from build123d import *

# Parameters (mm, degrees)
SKETCH013_W          = 32
SKETCH013_H          = 3
POCKET_DEPTH         = 6.001
POCKET_DEPTH_BACK    = -6.001
POCKET001_DEPTH      = 6.001
POCKET001_DEPTH_BACK = -6.001
POCKET002_DEPTH      = 6.001
POCKET002_DEPTH_BACK = -6.001


with BuildPart() as part:
    # AdditivePipe: sweep along a path in Sketch
    with BuildLine(Plane.XY) as additivepipe_path:
        ThreePointArc((0, 0), (-10.865453, 68.601773), (-42.398227, 130.488326))
    # Sketch002 → AdditivePipe (sweep)
    with BuildSketch(Plane.XZ):
        Polygon((-20, 6), (-20, -6), (-16, -6), (-16, -3), (-9, -3), (9, -3), (16, -3), (16, -6), (20, -6), (20, 6), (16, 6), (16, 3), (9, 3), (-9, 3), (-16, 3), (-16, 6), align=None)
    sweep(path=additivepipe_path.line)

    # AdditivePipe001: sweep along a path in Sketch001
    with BuildLine(Plane.XY) as additivepipe001_path:
        ThreePointArc((42.398227, 130.488326), (10.865453, 68.601773), (0, 0))
    # Sketch002 → AdditivePipe001 (sweep)
    with BuildSketch(Plane.XZ):
        Polygon((-20, 6), (-20, -6), (-16, -6), (-16, -3), (-9, -3), (9, -3), (16, -3), (16, -6), (20, -6), (20, 6), (16, 6), (16, 3), (9, 3), (-9, 3), (-16, 3), (-16, 6), align=None)
    sweep(path=additivepipe001_path.line)

    # SubtractivePipe: sweep along a path in Sketch
    with BuildLine(Plane.XY) as subtractivepipe_path:
        ThreePointArc((0, 0), (-10.865453, 68.601773), (-42.398227, 130.488326))
    # Sketch013 (on Face1 of AdditivePipe001) → SubtractivePipe (sweep, cut)
    with BuildSketch(Plane.XZ):
        with Locations((0, 4.5)):
            Rectangle(SKETCH013_W, SKETCH013_H)
    subtractivepipe = sweep(path=subtractivepipe_path.line, mode=Mode.SUBTRACT)

    # SubtractivePipe001: sweep along a path in Sketch001
    with BuildLine(Plane.XY) as subtractivepipe001_path:
        ThreePointArc((42.398227, 130.488326), (10.865453, 68.601773), (0, 0))
    # Sketch013 (on Face1 of AdditivePipe001) → SubtractivePipe001 (sweep, cut)
    with BuildSketch(Plane.XZ):
        with Locations((0, 4.5)):
            Rectangle(SKETCH013_W, SKETCH013_H)
    subtractivepipe001 = sweep(path=subtractivepipe001_path.line, mode=Mode.SUBTRACT)

    # Mirrored: SubtractivePipe across XY
    add(subtractivepipe.mirror(Plane.XY), mode=Mode.SUBTRACT)

    # Mirrored001: SubtractivePipe001 across XY
    add(subtractivepipe001.mirror(Plane.XY), mode=Mode.SUBTRACT)

    # Sketch007 → Pocket (cut, two sides)
    with BuildSketch(Plane.XY) as pocket_sk:
        with BuildLine():
            Line((-4.5, 0), (4.5, 0))
            Line((4.5, 0), (4.5, 7))
            ThreePointArc((4.5, 7), (0, 19.361903), (-4.5, 7))
            Line((-4.5, 0), (-4.5, 7))
        make_face()
    extrude(amount=-POCKET_DEPTH, mode=Mode.SUBTRACT)
    extrude(pocket_sk.sketch, amount=-POCKET_DEPTH_BACK, mode=Mode.SUBTRACT)

    # Sketch008 → Pocket001 (cut, two sides)
    with BuildSketch(Plane.XY) as pocket001_sk:
        with BuildLine():
            Line((-46.038804, 127.843292), (-38.757651, 133.13336))
            Line((-38.757651, 133.13336), (-34.643154, 127.470241))
            ThreePointArc((-41.924307, 122.180173), (-31.017586, 114.824218), (-34.643154, 127.470241))
            Line((-46.038804, 127.843292), (-41.924307, 122.180173))
        make_face()
    extrude(amount=-POCKET001_DEPTH, mode=Mode.SUBTRACT)
    extrude(pocket001_sk.sketch, amount=-POCKET001_DEPTH_BACK, mode=Mode.SUBTRACT)

    # Sketch009 → Pocket002 (cut, two sides)
    with BuildSketch(Plane.XY) as pocket002_sk:
        with BuildLine():
            Line((38.757651, 133.13336), (46.038804, 127.843292))
            Line((46.038804, 127.843292), (41.924307, 122.180173))
            ThreePointArc((34.643154, 127.470241), (31.017586, 114.824218), (41.924307, 122.180173))
            Line((38.757651, 133.13336), (34.643154, 127.470241))
        make_face()
    extrude(amount=-POCKET002_DEPTH, mode=Mode.SUBTRACT)
    extrude(pocket002_sk.sketch, amount=-POCKET002_DEPTH_BACK, mode=Mode.SUBTRACT)


solid = part.part
Input: part model. Units: mm. Frame: model coordinates. A direction names the side the tool comes from. Coordinates: 2 decimals unless noted, no trailing zeros. Order: outer loops, then holes, each group sorted by start corner. A loop starts at its lowest first (then second) coordinate and runs counter-clockwise, first axis right, second up. Notation, with made-up numbers: M 82.25,7.5 L 138.25,7.5 A6 ccw 138.25,14.5 Z; hole C -3,39.5 d4. An arc over 180 degrees is marked long. Answer as CSV lines item,"result".
1. Section B-B (x = -31). Return the cut outline in (y, z), then the cut area to 3 significant figures.
Reported:
outline,"M 65.75,-6 L 77.17,-6 L 77.17,-3 L 114.84,-3 L 114.84,3 L 77.17,3 L 77.17,6 L 65.75,6 Z; M 126.14,-3 L 138.77,-3 L 138.77,3 L 126.14,3 Z"
area,"439 mm2"
2. Section A-A (z = 4.5). Return the cut outline in (x, y), then the cut area to 3 significant figures.
Reported:
outline,"M -58.58,118.73 A202 cw -20,0 L -16,0 A206 ccw -55.34,121.08 Z; M -29.45,139.89 A238 cw 0,85.79 A238 cw 29.45,139.89 L 26.22,142.24 A242 ccw 0,96.33 A242 ccw -26.22,142.24 Z; M 16,0 L 20,0 A202 cw 58.58,118.73 L 55.34,121.08 A206 ccw Z"
area,"1,480 mm2"
3. Pull-direction query (X, two-part tool) for faces 1 (the cylindrical face through (-29.614, 61.576, -0.084)), 2 (the cylindrical face through (30.163, 63.266, 0.084)), 3 (the cylindrical face through (0.239, 19.358, 0.042)), 4 (the cylindrical face through (13.176, 114.178, -4.479)); classes: released by +X, released by -X, zero draft, split by the parting line, or undercut.
Reported:
face 1,"released by -X"
face 2,"released by +X"
face 3,"undercut"
face 4,"undercut"
4. Access query for faces 5 (the flat face through (4.5, 3, 0)), 6 (the cylindrical face through (26.364, 64.519, -4.521)), 7 (the cylindrical face through (13.176, 114.178, 4.521)), 8 (the cylindrical face through (-31.21, 114.69, 0.04)). Directions: +Z, -Z, +X, -X, +Y, -Y. A direction counts if a zero-diameter tool reaches every point of the face in a straight line with its end or side. Return the directions, or none.
Reported:
face 5,"+Z, -Z, -Y"
face 6,"-Z"
face 7,"+Z"
face 8,"+Z, -Z"
5. Section D-D (x = 22.5). Return the cut outline in (y, z), then the cut area to 3 significant figures.
Reported:
outline,"M 31.68,-6 L 51.34,-6 L 51.34,-3 L 129.78,-3 L 129.78,-6 L 136.98,-6 L 136.98,6 L 129.78,6 L 129.78,3 L 51.34,3 L 51.34,6 L 31.68,6 Z"
area,"793 mm2"
6. Section C-C (y = 112). Return the cut outline in (x, z).
Reported:
outline,"M -53.89,-6 L -49.11,-6 L -49.11,-3 L -12,-3 L -12,-6 L -7.48,-6 L -7.48,6 L -12,6 L -12,3 L -49.11,3 L -49.11,6 L -53.89,6 Z; M 7.48,-6 L 12,-6 L 12,-3 L 49.11,-3 L 49.11,-6 L 53.89,-6 L 53.89,6 L 49.11,6 L 49.11,3 L 12,3 L 12,6 L 7.48,6 Z"
7. Material intervals for line 1 (X direction, y = 125, z = -2.75); line 2 (Z direction, x = 16, y = 112.5); line 3 (X direction, y = 102.5, z = 1.75), sorted ascending. Write a range as from..to.
Reported:
line 1,"-49.95..-43.97, -29.78..-14.78, 14.78..29.78, 43.97..49.95"
line 2,"-3..3"
line 3,"-47.94..-2.78, 2.78..47.94"
8. First-contact query: P1, Ø11, axis at x = 35.13, y = 120.49, coming from the +Z side; P2, Ø2, axis at y = 89.5, z = -1, coming from the +X side; P3, Ø6, axis at x = 31, z = -4.5, coming from the +Y side; P4, Ø16, axis at x = 0, y = 12.36, coming from the -Z side. Flat tips, straight axial feed; report the tip coordinate or a pass-through.
Reported:
P1,"through"
P2,"x = 41.41"
P3,"y = 140.95"
P4,"z = -3"
